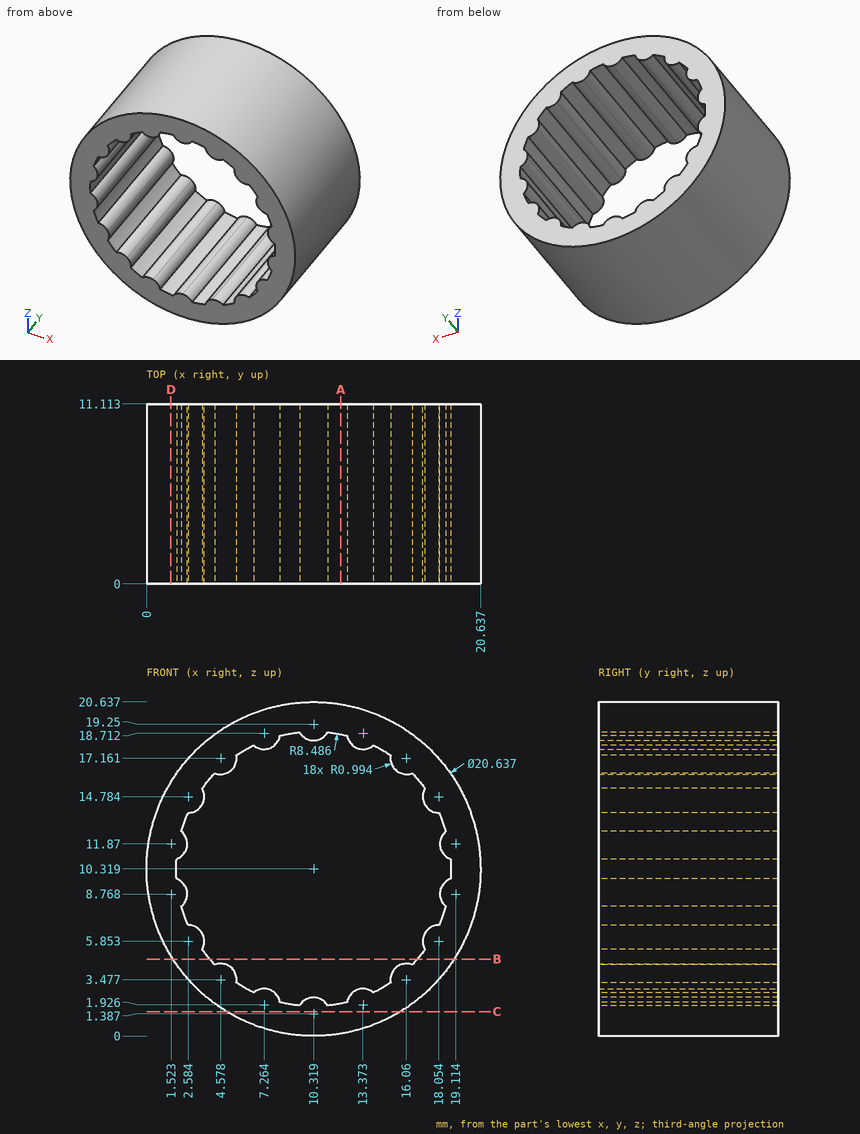
Here's the drawing with two shaded views (mm, measured from the low corner). I have some questions. Round coordinates to 2 decimals unless told otherwise and drop trailing zeros. Write each loop counter-clockwise with the first axis right and the second up, starting at its lowest first coordinate (ties: lowest second). Pieces come first, ordered by that corner, then holes. Notation, with made-up numbers: M 26.5,-38.75 L 35.5,-38.75 A30 ccw 35.5,-15.75 Z; hole C 59.5,72 d4. An arc over 180 degrees is marked long. Answer in a Markdown table with one row per item. Add a question column.
Q1. Will these pins go through, and if not, where does the flat tip stop? pin 1 Ø6 at (y, z) = (3, 14.5) entering from +X; pin 2 Ø5 at (y, z) = (9.5, 16) entering from -X.
Q2. Imagine slicing it at B-B (z = 4.75). Please give me the cut outline in (x, y) (1 decimal).
Q3. Imagine slicing it at A-A (x = 12). Please give me the cut outline in (y, z).
Q4. Imagine slicing it at D-D (x = 1.5). Please give me the cut outline in (y, z).
Q5. If I drill on line 1 (Z direction, x = 10.25, y = 8.5); line 2 (Z direction, x = 16.25, y = 2.25) (1 decimal); line 3 (X direction, y = 5.75, z = 7.25), over which ranges is the centre line in solid material (lowest first)? Write a range as from..to.
Q6. Imagine slicing it at C-C (z = 1.5). Please give me the cut outline in (x, y), then the cut area to 3 significant figures.
Values:
| question | item | result |
|---|---|---|
| 1 | pin 1 | x = 20.57 |
| 1 | pin 2 | x = 0.5 |
| 2 | outline | M 1.6,0 L 3.9,0 L 3.9,11.1 L 1.6,11.1 Z; M 16.7,0 L 19,0 L 19,11.1 L 16.7,11.1 Z |
| 3 | outline | M 0,0.14 L 11.11,0.14 L 11.11,2 L 0,2 Z; M 0,18.64 L 11.11,18.64 L 11.11,20.5 L 0,20.5 Z |
| 4 | outline | M 0,4.96 L 11.11,4.96 L 11.11,15.68 L 0,15.68 Z |
| 5 | line 1 | 0..2.38, 18.26..20.64 |
| 5 | line 2 | 1.9..4.5, 16.2..18.8 |
| 5 | line 3 | 0.47..2.41, 18.23..20.17 |
| 6 | outline | M 4.96,0 L 15.68,0 L 15.68,11.11 L 4.96,11.11 Z |
| 6 | area | 119 mm^2 |
